The listing builds one solid part. Answer for the finished solid, in the listing's coordinates (mm). Face numbers are marked on the shaded views. A direction names the side the tool comes from. Round coordinates to 2 decimals unless told otherwise and drop trailing zeros. Order: outer loops, then holes, each group sorted by start corner. A loop starts at its lowest first (then second) coordinate and runs counter-clockwise, first axis right, second up. Notation, with made-up numbers: M -12,-8.75 L -5,-8.75 A31 ccw -5,24.25 Z; hole C 43,49.25 d6. An arc over 180 degrees is marked long. Write item = value, one per line. Start each with the question number.
(1) A cutting plane is placed at C-C, the plane z = 10. Count the separate pieces of the cut face and the enclosed holes in it, and give its area (3 significant figures).
(2) A cutting plane is placed at B-B, the plane x = 0. Determine the outline of the cut face in (y, z).
(3) For a pull along X with two mould halves and no side action, classify the marked faces 6, 7 and 8 as released by +X, released by -X, zero draft, split by the parting line, or undercut.
(4) Which of the six approach directions +Z, -Z, +X, -X, +Y, -Y give full straight-line access (tool end or side, diameter ignored) to the marked faces 1, 2, 3, 4 and 5?
(5) A cutting plane is placed at D-D, the plane x = -11.5. Determine the outline of the cut face in (y, z).
(6) Straight lines are drawn through the part: probe 1 along Y at (x, z) = (3.75, 10.75); probe 2 along Y at (x, z) = (-4.25, 8.5); probe 3 along Y at (x, z) = (5, 5) (3 decimals). For each, find the intervals that lie inside material, in ascending order. Write a range as from..to.
(7) A cutting plane is placed at A-A, the plane y = -7.5. Determine the outline of the cut face in (x, z).
(8) Each of these flat-tipped pins is pushed along its axis until it touches: pin 1 (1.5 mm diameter, centred on y = 11.5, z = 3.5, fed in from +X); pin 2 (4.5 mm diameter, centred on x = -14.25, y = 9.5, fed in from -Z); pin 3 (1 mm diameter, centred on x = 3, y = 2, fed in from -Z); pin 4 (5 mm diameter, centred on x = -1, y = -6.5, fed in from +Z). Where does it stop, or does it pass through?
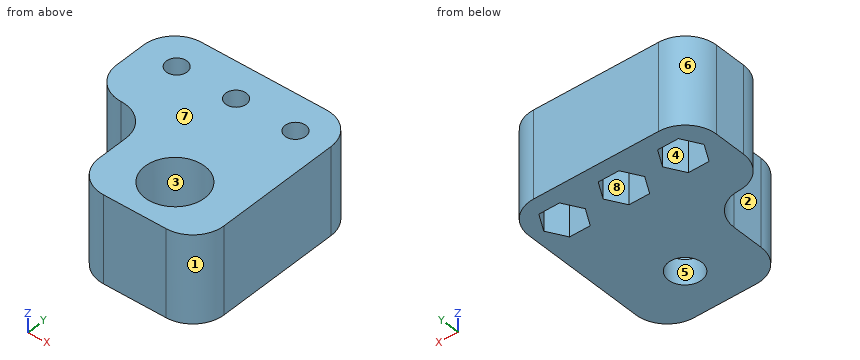
from build123d import *

# Parameters (mm, degrees)
F0_W      = 20
F0_H      = 30
F1_DEPTH  = 14
F2_R      = 2.65
F3_DEPTH  = 14.001
F4_R      = 1.65
F5_DEPTH  = 14.001
F6_W      = 15
F6_H      = 14
F7_DEPTH  = 10
F8_R      = 1.65
F9_DEPTH  = 14.001
F10_R     = 4.99999
F12_DEPTH = 8
F13_R     = 4.75
F14_DEPTH = 10


# Not quite as in the source:
# - a fillet or chamfer is up to 0.001 mm smaller than in the source, because OpenCascade refuses the exact size


with BuildPart() as f1:
    # F0 (on Top) → F1 (new body)
    with BuildSketch(Plane.XY):
        Rectangle(F0_W, F0_H)
    extrude(amount=F1_DEPTH)

    # F2 (on face) → F3 (cut, through all)
    with BuildSketch(Plane.XY.offset(14)):
        with Locations((0, -7.5)):
            Circle(F2_R)
    extrude(amount=-F3_DEPTH, mode=Mode.SUBTRACT)

    # F4 (on face) → F5 (cut, through all)
    with BuildSketch(Plane.XY.offset(14)):
        with Locations((-4.75, 9.5)):
            Circle(F4_R)
        with Locations((4.75, 9.5)):
            Circle(F4_R)
    extrude(amount=-F5_DEPTH, mode=Mode.SUBTRACT)

    # F6 (on face) → F7 (join)
    with BuildSketch(Plane(origin=(-10, 0, 0), x_dir=(0, -1, 0), z_dir=(-1, 0, 0))):
        with Locations((-7.5, 7)):
            Rectangle(F6_W, F6_H)
    extrude(amount=F7_DEPTH)

    # F8 (on face) → F9 (cut, through all)
    with BuildSketch(Plane.XY.offset(14)):
        with Locations((-14.25, 9.5)):
            Circle(F8_R)
    extrude(amount=-F9_DEPTH, mode=Mode.SUBTRACT)

    # F10 (radius 5 in the source; OpenCascade refuses exactly that, so slightly less here)
    f10_edges = [f1.edges().sort_by_distance(p)[0] for p in [
        (-12.6, 9.5, 7),
        (-10, -15, 7),
        (10, -15, 7),
        (-10, 0, 7),
        (-20, 0, 7),
        (-20, 15, 7),
        (10, 15, 7),
    ]]
    fillet(f10_edges, radius=F10_R)

    # F11 (on face) → F12 (cut)
    with BuildSketch(Plane(origin=(0, 0, 0), x_dir=(1, 0, 0), z_dir=(0, 0, -1))):
        Polygon((-17.5697640478, -9.5), (-15.9098820239, -12.375), (-12.5901179761, -12.375), (-10.9302359522, -9.5), (-12.5901179761, -6.625), (-15.9098820239, -6.625), align=None)
        Polygon((3.0901179761, -6.625), (1.4302359522, -9.5), (3.0901179761, -12.375), (6.4098820239, -12.375), (8.0697640478, -9.5), (6.4098820239, -6.625), align=None)
        Polygon((-6.4098820239, -6.625), (-8.0697640478, -9.5), (-6.4098820239, -12.375), (-3.0901179761, -12.375), (-1.4302359522, -9.5), (-3.0901179761, -6.625), align=None)
    extrude(amount=-F12_DEPTH, mode=Mode.SUBTRACT)

    # F13 (on face) → F14 (cut)
    with BuildSketch(Plane.XY.offset(14)):
        with Locations((0, -7.5)):
            Circle(F13_R)
    extrude(amount=-F14_DEPTH, mode=Mode.SUBTRACT)


solid = f1.part
Reported:
q1.separate_pieces = 1
q1.enclosed_holes = 4
q1.area = 632 mm²
q2.outline = M -15,0 L -10.15,0 L -10.15,4 L -12.25,4 L -12.25,14 L -15,14 Z; M -4.85,0 L 15,0 L 15,14 L -2.75,14 L -2.75,4 L -4.85,4 Z
q3.face_6 = released by -X
q3.face_7 = zero draft
q3.face_8 = undercut
q4.face_1 = +Z, -Z, +X, -Y
q4.face_2 = +Z, -Z, -X, -Y
q4.face_3 = +Z
q4.face_4 = -Z
q4.face_5 = +Z, -Z
q5.outline = M -1.43,0 L 8.51,0 L 8.51,8 L 10.49,8 L 10.49,0 L 15,0 L 15,14 L -1.43,14 Z
q6.probe_1 = -15..-10.42, -4.58..8.19, 10.81..15
q6.probe_2 = -15..-9.62, -5.38..7.93, 11.07..15
q6.probe_3 = -15..6.625, 12.375..15
q7.outline = M -10,0 L -2.65,0 L -2.65,4 L -4.75,4 L -4.75,14 L -10,14 Z; M 2.65,0 L 10,0 L 10,14 L 4.75,14 L 4.75,4 L 2.65,4 Z
q8.pin_1 = 9.94
q8.pin_2 = 8
q8.pin_3 = 0
q8.pin_4 = 4
